from build123d import *

# Parameters (mm, degrees)
SKETCH1_R                     = 125
BOSS_EXTRUDE1_DEPTH           = 10
SKETCH2_R                     = 5
SKETCH2_R_2                   = 32
SKETCH2_R_3                   = 5.5
CUT_EXTRUDE1_DEPTH            = 10
CHAMFER1_SIZE                 = 3
CHAMFER2_SIZE                 = 3
CHAMFER2_SIZE2                = 8.242432258
CIRPATTERN1_COUNT             = 2
CHAMFER1_OF_CIRPATTERN1_SIZE  = 3
CHAMFER2_OF_CIRPATTERN1_SIZE2 = 8.242432258
CHAMFER2_OF_CIRPATTERN1_SIZE  = 3


with BuildPart() as part:
    # Sketch1 → Boss-Extrude1 (new body)
    with BuildSketch(Plane.XY):
        Circle(SKETCH1_R)
    extrude(amount=BOSS_EXTRUDE1_DEPTH)

    # Sketch2 → Cut-Extrude1 (cut)
    with BuildSketch(Plane(origin=(0, 0, 0), x_dir=(-1, 0, 0), z_dir=(0, 0, -1))):
        Circle(SKETCH2_R)
        with Locations((-47.877777695, -40.174225605)):
            Circle(SKETCH2_R_2)
        with Locations((10.853011104, -61.550484563)):
            Circle(SKETCH2_R_3)
        with Locations((40.174225605, -47.877777695)):
            Circle(SKETCH2_R_3)
        with Locations((58.730788799, -21.376258958)):
            Circle(SKETCH2_R_3)
    cut_extrude1 = extrude(amount=-CUT_EXTRUDE1_DEPTH, mode=Mode.SUBTRACT)

    # Chamfer1
    chamfer1_edges = [part.edges().sort_by_distance(p)[0] for p in [
        (79.877777695, -40.174225605, 0),
    ]]
    chamfer(chamfer1_edges, length=CHAMFER1_SIZE)

    # Chamfer2
    chamfer2_edges = [part.edges().sort_by_distance(p)[0] for p in [
        (-5.353011104, -61.550484563, 0),
        (-34.674225605, -47.877777695, 0),
        (-53.230788799, -21.376258958, 0),
    ]]
    chamfer2_side = [part.faces().sort_by_distance(p)[0] for p in [
        (-3.873503852, 3.722299955, 0),
    ]]
    chamfer(chamfer2_edges, length=CHAMFER2_SIZE, length2=CHAMFER2_SIZE2, reference=chamfer2_side[0])

    # CirPattern1: Cut-Extrude1 ×2 about axis
    cirpattern1_axis = Axis((0, 0, 0), (0, 0, 1))
    for i in range(1, CIRPATTERN1_COUNT):
        add(cut_extrude1.rotate(cirpattern1_axis, i * 360 / CIRPATTERN1_COUNT), mode=Mode.SUBTRACT)

    # Chamfer1 of CirPattern1
    chamfer1_of_cirpattern1_edges = [part.edges().sort_by_distance(p)[0] for p in [
        (-79.877777695, 40.174225605, 0),
    ]]
    chamfer(chamfer1_of_cirpattern1_edges, length=CHAMFER1_OF_CIRPATTERN1_SIZE)

    # Chamfer2 of CirPattern1
    chamfer2_of_cirpattern1_edges = [part.edges().sort_by_distance(p)[0] for p in [
        (5.353011104, 61.550484563, 0),
        (34.674225605, 47.877777695, 0),
        (53.230788799, 21.376258958, 0),
    ]]
    chamfer(chamfer2_of_cirpattern1_edges, length=CHAMFER2_OF_CIRPATTERN1_SIZE, length2=CHAMFER2_OF_CIRPATTERN1_SIZE2)


solid = part.part
Read the model definition and answer for the solid it produces. Units are mm, in the model's axes. Coordinates: 2 decimals unless noted, no trailing zeros. Write each loop counter-clockwise with the first axis right and the second up, starting at its lowest first coordinate (ties: lowest second). Pieces come first, ordered by that corner, then holes. Notation, with made-up numbers: (49.5, -31) - (61.5, -31) arc R26 cw to (61.5, -10) - close; hole circle Ø3 at (-34, 74). An arc over 180 degrees is marked (long way). One line per question, with ' | ' between items.
Q1. Find section B-B, the plane z = 5.5. State how many separate pieces and enclosed holes the cut face has, plus the area to 3 significant figures.
Result set:
separate pieces: 1 | enclosed holes: 9 | area: 41,800 mm^2
Q2. Find section A-A, the plane y = 0. Write down the section's boundary in (x, z), plus the area to 3 significant figures.
Result set:
outline: (-125, 0) - (-5, 0) - (-5, 10) - (-125, 10) - close; (5, 0) - (125, 0) - (125, 10) - (5, 10) - close | area: 2,400 mm^2
Q3. Determine the mould class of faces 1 (the flat face through (26, 2, 0)), 2 (the cylindrical face through (-124.88, 5.5, 4.93)), 3 (the conical face through (-79.992, 38.761, 2.854)) for opening direction Y: +Y half, -Y half, draft (parallel to the pull), parting line (faces both ways), or undercut.
Result set:
face 1: draft | face 2: parting line | face 3: undercut
Q4. Consider L1, parallel to Y at x = 0, z = 3.75; L2, parallel to X at y = -66.5, z = 6.25; L3, parallel to Y at x = 41.5, z = 9.5. Determine where each line is inside the solid, lowest interval first. Write a range as [from, to].
Result set:
L1: [-125, -5], [5, 125] | L2: [-105.84, -14.63], [-7.08, 29.69], [66.07, 105.84] | L3: [-117.91, -71.53], [-8.82, 42.54], [53.22, 117.91]
Q5. Find section D-D, the plane y = -102. Write down the section's boundary in (x, z).
Result set:
outline: (-72.26, 0) - (72.26, 0) - (72.26, 10) - (-72.26, 10) - close
Q6. Each of these flat-tipped pins is pushed along its axis until it touches: P1, Ø1, axis at x = -97.5, z = 8.5, coming from the -Y side; P2, Ø12.5, axis at x = -10.85, y = -61.55, coming from the +Z side; P3, Ø5, axis at y = -43.5, z = 3.5, coming from the -X side; P4, Ø1.5, axis at x = -77, z = 2, coming from the -Y side. Where does it stop, or does it pass through?
Result set:
P1: y = -78.84 | P2: z = 10 | P3: x = -118.08 | P4: y = -99.05
